Source: CAD feature listing. Evaluate the final solid. Frame: model axes, mm. A direction names the side the tool comes from. Round coordinates to 2 decimals unless told otherwise and drop trailing zeros. Order: outer loops, then holes, each group sorted by start corner. A loop starts at its lowest first (then second) coordinate and runs counter-clockwise, first axis right, second up. Notation, with made-up numbers: (-14.5, 23.25) -> (29.5, 23.25) arc R21 ccw to (29.5, 36.25) -> close; hole circle Ø2 at (79, -2.75). An arc over 180 degrees is marked (long way). Answer as CSV lines item,"result". Start each with the question number.
(1) Set-up query: faces 1 (the flat face through (4, -36, 5.26)), 2 (the cylindrical face through (3.63, -33.36, 4.21)), 3 (the cylindrical face through (9.21, -13.52, 1.03)). Return all of +Z, -Z, +X, -X, +Y, -Y with unobstructed straight access to the full face (end or side cutting, diameter ignored); none if empty.
(2) Section query B-B (y = -19.87). Output: boundary loops of the cut face in (x, z).
(3) Contact query for flat-ended pins moving along their axis: P1, Ø5, axis at x = 7.95, y = -15.938, coming from the +Z side; P2, Ø3.5, axis at x = 7.95, y = -31.762, coming from the -Z side. Output: stop coordinate, or through.
(4) Section query A-A (z = 3.6). Count the separate pieces of the cut face and the enclosed holes in it, plus the area to 3 significant figures.
(5) Line query: line 1 along X through (y, z) = (-43.5, 1.5); line 2 along Y through (x, z) = (12, 0.8); line 3 along Y through (x, z) = (1.75, 4.85). Output: solid intervals per line, ascending. Write a range as from..to.
(6) Section query D-D (y = -31). Output: boundary loops of the cut face in (x, z), plus the area to 3 significant figures.
```python
from build123d import *

# Parameters (mm, degrees)
F0_W     = 15.9
F0_H     = 47.7
F0_R     = 2.45
F1_DEPTH = 3.18
F2_DEPTH = 5.26
F3_W     = 12.9
F3_H     = 44.7
F3_R     = 3.225
F3_R_2   = 2.725
F4_DEPTH = 2.08


with BuildPart() as f1:
    # F0 (on Top) → F1 (new body)
    with BuildSketch(Plane.XY):
        with Locations((7.95, -23.85)):
            Rectangle(F0_W, F0_H)
        with Locations((3.95, -43.75)):
            Circle(F0_R, mode=Mode.SUBTRACT)
        with Locations((3.95, -35.79)):
            Circle(F0_R, mode=Mode.SUBTRACT)
        with Locations((3.95, -27.83)):
            Circle(F0_R, mode=Mode.SUBTRACT)
        with Locations((11.95, -43.75)):
            Circle(F0_R, mode=Mode.SUBTRACT)
        with Locations((11.95, -35.79)):
            Circle(F0_R, mode=Mode.SUBTRACT)
        with Locations((11.95, -27.83)):
            Circle(F0_R, mode=Mode.SUBTRACT)
        with Locations((3.95, -19.87)):
            Circle(F0_R, mode=Mode.SUBTRACT)
        with Locations((3.95, -11.91)):
            Circle(F0_R, mode=Mode.SUBTRACT)
        with Locations((3.95, -3.95)):
            Circle(F0_R, mode=Mode.SUBTRACT)
        with Locations((11.95, -19.87)):
            Circle(F0_R, mode=Mode.SUBTRACT)
        with Locations((11.95, -11.91)):
            Circle(F0_R, mode=Mode.SUBTRACT)
        with Locations((11.95, -3.95)):
            Circle(F0_R, mode=Mode.SUBTRACT)
    extrude(amount=F1_DEPTH)

    # F0 (on Top) → F2 (join)
    with BuildSketch(Plane.XY):
        with Locations((3.95, -3.95)):
            Circle(F0_R)
        with Locations((11.95, -3.95)):
            Circle(F0_R)
        with Locations((11.95, -11.91)):
            Circle(F0_R)
        with Locations((3.95, -11.91)):
            Circle(F0_R)
        with Locations((3.95, -19.87)):
            Circle(F0_R)
        with Locations((11.95, -19.87)):
            Circle(F0_R)
        with Locations((11.95, -27.83)):
            Circle(F0_R)
        with Locations((3.95, -27.83)):
            Circle(F0_R)
        with Locations((3.95, -35.79)):
            Circle(F0_R)
        with Locations((11.95, -35.79)):
            Circle(F0_R)
        with Locations((11.95, -43.75)):
            Circle(F0_R)
        with Locations((3.95, -43.75)):
            Circle(F0_R)
    extrude(amount=F2_DEPTH)

    # F3 (on face) → F4 (cut)
    with BuildSketch(Plane(origin=(0, 0, 0), x_dir=(1, 0, 0), z_dir=(0, 0, -1))):
        with Locations((7.95, 23.85)):
            Rectangle(F3_W, F3_H)
        with Locations((7.95, 8.025)):
            Circle(F3_R, mode=Mode.SUBTRACT)
        with Locations((7.95, 15.938)):
            Circle(F3_R, mode=Mode.SUBTRACT)
        with Locations((7.95, 23.85)):
            Circle(F3_R, mode=Mode.SUBTRACT)
        with Locations((7.95, 31.762)):
            Circle(F3_R, mode=Mode.SUBTRACT)
        with Locations((7.95, 39.675)):
            Circle(F3_R, mode=Mode.SUBTRACT)
        with Locations((7.95, 39.675)):
            Circle(F3_R_2)
        with Locations((7.95, 31.762)):
            Circle(F3_R_2)
        with Locations((7.95, 23.85)):
            Circle(F3_R_2)
        with Locations((7.95, 15.938)):
            Circle(F3_R_2)
        with Locations((7.95, 8.025)):
            Circle(F3_R_2)
    extrude(amount=-F4_DEPTH, mode=Mode.SUBTRACT)


solid = f1.part
```
Answer block:
1,face 1,"+Z, +X, -X, +Y, -Y"
1,face 2,"+Z"
1,face 3,"-Z"
2,outline,"(0, 0) -> (1.5, 0) -> (1.5, 2.08) -> (14.4, 2.08) -> (14.4, 0) -> (15.9, 0) -> (15.9, 3.18) -> (14.4, 3.18) -> (14.4, 5.26) -> (9.5, 5.26) -> (9.5, 3.18) -> (6.4, 3.18) -> (6.4, 5.26) -> (1.5, 5.26) -> (1.5, 3.18) -> (0, 3.18) -> close"
3,P1,"z = 3.18"
3,P2,"z = 2.08"
4,separate pieces,"12"
4,enclosed holes,"0"
4,area,"226 mm2"
5,line 1,"0..1.5, 14.4..15.9"
5,line 2,"-47.7..-46.2, -1.5..0"
5,line 3,"-44.83..-42.67, -36.87..-34.71, -28.91..-26.75, -20.95..-18.79, -12.99..-10.83, -5.03..-2.87"
6,outline,"(0, 0) -> (1.5, 0) -> (1.5, 2.08) -> (4.82, 2.08) -> (4.82, 0) -> (5.33, 0) -> (5.33, 2.08) -> (10.57, 2.08) -> (10.57, 0) -> (11.08, 0) -> (11.08, 2.08) -> (14.4, 2.08) -> (14.4, 0) -> (15.9, 0) -> (15.9, 3.18) -> (0, 3.18) -> close"
6,area,"25.9 mm2"
